```python
from build123d import *

# Parameters (mm, degrees)
F0_R     = 15
F1_DEPTH = 1.5
F2_DEPTH = 6.8


with BuildPart() as f1:
    # F0 (on Top) → F1 (new body)
    with BuildSketch(Plane.XY):
        with BuildLine():
            ThreePointArc((24.1652138662, -4.8646622494), (24.5285040494, -2.4443790825), (24.65, 0))
            ThreePointArc((24.65, 0), (18.0037803541, 16.8370541652), (1.6490756219, 24.5947768763))
            ThreePointArc((1.6490756219, 24.5947768763), (0, 23), (-1.6490756219, 24.5947768763))
            ThreePointArc((-1.6490756219, 24.5947768763), (-17.4301821562, 17.4301821562), (-24.5947768763, 1.6490756219))
            ThreePointArc((-24.5947768763, 1.6490756219), (-23.4639101733, 1.1470357113), (-23, 0))
            ThreePointArc((-23, 0), (-23.4639101733, -1.1470357113), (-24.5947768763, -1.6490756219))
            ThreePointArc((-24.5947768763, -1.6490756219), (-17.9529932576, -16.8911969112), (-3.1435634706, -24.4487322515))
            ThreePointArc((-3.1435634706, -24.4487322515), (0, -21.5), (3.1435634706, -24.4487322515))
            Line((3.1435634706, -24.4487322515), (12.969203616, -16.0692954907))
            ThreePointArc((12.969203616, -16.0692954907), (-18.6311104697, 8.9052918349), (20.65, 0))
            ThreePointArc((20.65, 0), (19.4738226895, -6.8696964896), (16.0792755585, -12.9568282197))
            Line((16.0792755585, -12.9568282197), (24.1652138662, -4.8646622494))
        make_face()
        with BuildLine():
            ThreePointArc((1.6490756219, 24.5947768763), (18.0037803541, 16.8370541652), (24.65, 0))
            ThreePointArc((24.65, 0), (24.5285040494, -2.4443790825), (24.1652138662, -4.8646622494))
            Line((24.1652138662, -4.8646622494), (27.771636901, -1.2554616043))
            ThreePointArc((27.771636901, -1.2554616043), (27.7929083207, -0.6278909749), (27.8, 0))
            ThreePointArc((27.8, 0), (25.6818028962, 10.6435426433), (19.65, 19.6651341211))
            ThreePointArc((19.65, 19.6651341211), (-25.6858981613, 10.6336557988), (7.1e-09, -27.8))
            ThreePointArc((7.1e-09, -27.8), (-2.2974435124, -26.8050529709), (-3.1435634706, -24.4487322515))
            ThreePointArc((-3.1435634706, -24.4487322515), (-17.9529932576, -16.8911969112), (-24.5947768763, -1.6490756219))
            ThreePointArc((-24.5947768763, -1.6490756219), (-26.3, 0), (-24.5947768763, 1.6490756219))
            ThreePointArc((-24.5947768763, 1.6490756219), (-17.4301821562, 17.4301821562), (-1.6490756219, 24.5947768763))
            ThreePointArc((-1.6490756219, 24.5947768763), (-0.0276154299, 26.2997688893), (1.65, 24.65))
            ThreePointArc((1.65, 24.65), (1.6497688893, 24.6223845701), (1.6490756219, 24.5947768763))
        make_face()
        with BuildLine():
            ThreePointArc((3.15, -24.65), (3.1483904564, -24.549314679), (3.1435634706, -24.4487322515))
            ThreePointArc((3.1435634706, -24.4487322515), (2.3974318813, -24.5331371898), (1.6490756219, -24.5947768763))
            ThreePointArc((1.6490756219, -24.5947768763), (1.6497688893, -24.6223845701), (1.65, -24.65))
            ThreePointArc((1.65, -24.65), (-0.0276154299, -26.2997688893), (-1.6490756219, -24.5947768763))
            ThreePointArc((-1.6490756219, -24.5947768763), (-2.3974318813, -24.5331371898), (-3.1435634706, -24.4487322515))
            ThreePointArc((-3.1435634706, -24.4487322515), (-2.2974435124, -26.8050529709), (7.1e-09, -27.8))
            ThreePointArc((7.1e-09, -27.8), (2.2273863633, -26.8773863582), (3.15, -24.65))
        make_face()
        with BuildLine():
            ThreePointArc((1.6490756219, -24.5947768763), (2.3974318813, -24.5331371898), (3.1435634706, -24.4487322515))
            ThreePointArc((3.1435634706, -24.4487322515), (0, -21.5), (-3.1435634706, -24.4487322515))
            ThreePointArc((-3.1435634706, -24.4487322515), (-2.3974318813, -24.5331371898), (-1.6490756219, -24.5947768763))
            ThreePointArc((-1.6490756219, -24.5947768763), (0, -23), (1.6490756219, -24.5947768763))
        make_face()
        with BuildLine():
            Line((12.969203616, -16.0692954907), (16.0792755585, -12.9568282197))
            ThreePointArc((16.0792755585, -12.9568282197), (19.4738226895, -6.8696964896), (20.65, 0))
            ThreePointArc((20.65, 0), (-18.6311104697, 8.9052918349), (12.969203616, -16.0692954907))
        make_face()
        Circle(F0_R, mode=Mode.SUBTRACT)
        with BuildLine():
            ThreePointArc((27.8, 0), (27.7929083207, -0.6278909749), (27.771636901, -1.2554616043))
            Line((27.771636901, -1.2554616043), (34.1742395873, 5.1520722659))
            Line((34.1742395873, 5.1520722659), (19.65, 19.6651341211))
            ThreePointArc((19.65, 19.6651341211), (25.6818028962, 10.6435426433), (27.8, 0))
        make_face()
    extrude(amount=-F1_DEPTH)

    # F0 (on Top) → F2 (join)
    with BuildSketch(Plane.XY):
        with BuildLine():
            ThreePointArc((24.1652138662, -4.8646622494), (24.5285040494, -2.4443790825), (24.65, 0))
            ThreePointArc((24.65, 0), (18.0037803541, 16.8370541652), (1.6490756219, 24.5947768763))
            ThreePointArc((1.6490756219, 24.5947768763), (0, 23), (-1.6490756219, 24.5947768763))
            ThreePointArc((-1.6490756219, 24.5947768763), (-17.4301821562, 17.4301821562), (-24.5947768763, 1.6490756219))
            ThreePointArc((-24.5947768763, 1.6490756219), (-23.4639101733, 1.1470357113), (-23, 0))
            ThreePointArc((-23, 0), (-23.4639101733, -1.1470357113), (-24.5947768763, -1.6490756219))
            ThreePointArc((-24.5947768763, -1.6490756219), (-17.9529932576, -16.8911969112), (-3.1435634706, -24.4487322515))
            ThreePointArc((-3.1435634706, -24.4487322515), (0, -21.5), (3.1435634706, -24.4487322515))
            Line((3.1435634706, -24.4487322515), (12.969203616, -16.0692954907))
            ThreePointArc((12.969203616, -16.0692954907), (-18.6311104697, 8.9052918349), (20.65, 0))
            ThreePointArc((20.65, 0), (19.4738226895, -6.8696964896), (16.0792755585, -12.9568282197))
            Line((16.0792755585, -12.9568282197), (24.1652138662, -4.8646622494))
        make_face()
        with BuildLine():
            ThreePointArc((1.6490756219, 24.5947768763), (18.0037803541, 16.8370541652), (24.65, 0))
            ThreePointArc((24.65, 0), (24.5285040494, -2.4443790825), (24.1652138662, -4.8646622494))
            Line((24.1652138662, -4.8646622494), (27.771636901, -1.2554616043))
            ThreePointArc((27.771636901, -1.2554616043), (27.7929083207, -0.6278909749), (27.8, 0))
            ThreePointArc((27.8, 0), (25.6818028962, 10.6435426433), (19.65, 19.6651341211))
            ThreePointArc((19.65, 19.6651341211), (-25.6858981613, 10.6336557988), (7.1e-09, -27.8))
            ThreePointArc((7.1e-09, -27.8), (-2.2974435124, -26.8050529709), (-3.1435634706, -24.4487322515))
            ThreePointArc((-3.1435634706, -24.4487322515), (-17.9529932576, -16.8911969112), (-24.5947768763, -1.6490756219))
            ThreePointArc((-24.5947768763, -1.6490756219), (-26.3, 0), (-24.5947768763, 1.6490756219))
            ThreePointArc((-24.5947768763, 1.6490756219), (-17.4301821562, 17.4301821562), (-1.6490756219, 24.5947768763))
            ThreePointArc((-1.6490756219, 24.5947768763), (-0.0276154299, 26.2997688893), (1.65, 24.65))
            ThreePointArc((1.65, 24.65), (1.6497688893, 24.6223845701), (1.6490756219, 24.5947768763))
        make_face()
        with BuildLine():
            ThreePointArc((3.15, -24.65), (3.1483904564, -24.549314679), (3.1435634706, -24.4487322515))
            ThreePointArc((3.1435634706, -24.4487322515), (2.3974318813, -24.5331371898), (1.6490756219, -24.5947768763))
            ThreePointArc((1.6490756219, -24.5947768763), (1.6497688893, -24.6223845701), (1.65, -24.65))
            ThreePointArc((1.65, -24.65), (-0.0276154299, -26.2997688893), (-1.6490756219, -24.5947768763))
            ThreePointArc((-1.6490756219, -24.5947768763), (-2.3974318813, -24.5331371898), (-3.1435634706, -24.4487322515))
            ThreePointArc((-3.1435634706, -24.4487322515), (-2.2974435124, -26.8050529709), (7.1e-09, -27.8))
            ThreePointArc((7.1e-09, -27.8), (2.2273863633, -26.8773863582), (3.15, -24.65))
        make_face()
        with BuildLine():
            ThreePointArc((1.6490756219, -24.5947768763), (2.3974318813, -24.5331371898), (3.1435634706, -24.4487322515))
            ThreePointArc((3.1435634706, -24.4487322515), (0, -21.5), (-3.1435634706, -24.4487322515))
            ThreePointArc((-3.1435634706, -24.4487322515), (-2.3974318813, -24.5331371898), (-1.6490756219, -24.5947768763))
            ThreePointArc((-1.6490756219, -24.5947768763), (0, -23), (1.6490756219, -24.5947768763))
        make_face()
        with BuildLine():
            ThreePointArc((27.8, 0), (27.7929083207, -0.6278909749), (27.771636901, -1.2554616043))
            Line((27.771636901, -1.2554616043), (34.1742395873, 5.1520722659))
            Line((34.1742395873, 5.1520722659), (19.65, 19.6651341211))
            ThreePointArc((19.65, 19.6651341211), (25.6818028962, 10.6435426433), (27.8, 0))
        make_face()
    extrude(amount=F2_DEPTH)


solid = f1.part
```
Input: part model. Units: mm. Frame: model coordinates. Give positions to 0.01 mm unless a question says otherwise; leave off trailing zeros. Order: outer loops, then holes, each group sorted by start corner. A loop starts at its lowest first (then second) coordinate and runs counter-clockwise, first axis right, second up. Notation, with made-up numbers: M -2.75,64.25 L 19.25,64.25 A21 cw 19.25,81.25 Z; hole C -37.75,19 d3. An arc over 180 degrees is marked long. Return JSON: item names as keys, results as strings.
Item 1: Cut plane D-D (y = 17). Return loops of the section in (x, z), then the cut area to 3 significant figures.
Solutions:
{"outline": "M -22,-1.5 L 22.32,-1.5 L 22.32,6.8 L 11.72,6.8 L 11.72,0 L -11.72,0 L -11.72,6.8 L -22,6.8 Z", "area": "208 mm^2"}
Item 2: Cut plane A-A (z = 5.5). Return loops of the section in (x, y), then the cut area to 3 significant figures.
Solutions:
{"outline": "M 0,-27.8 A3.15 ccw 3.14,-24.45 L 12.97,-16.07 A20.65 cw long 16.08,-12.96 L 34.17,5.15 L 19.65,19.67 A27.8 ccw long Z; hole C -24.65,0 d3.3; hole C 0,-24.65 d3.3; hole C 0,24.65 d3.3", "area": "926 mm^2"}
Item 3: Pull-direction query (Y, two-part tool) for faces 1 (the cylindrical face through (-14.985, 0.66, -0.74)), 2 (the cylindrical face through (-25.4, 11.3, 2.6)), 3 (the flat face through (14, 6, 0)), 4 (the flat face through (7.988, -20.318, 2.592)); classes: +Y half, -Y half, draft (parallel to the pull), parting line (faces both ways), or undercut.
Solutions:
{"face 1": "undercut", "face 2": "parting line", "face 3": "undercut", "face 4": "-Y half"}
Item 4: First-contact query: P1, Ø5, axis at x = -6.5, y = 13, coming from the +Z side; P2, Ø18, axis at x = 0, y = 0, coming from the +Z side; P3, Ø1, axis at x = 7, z = 0, coming from the +Y side; P4, Ø2, axis at y = 18.5, z = 3.5, coming from the -X side. Flat tips, straight axial feed; report the tip coordinate or a pass-through.
Solutions:
{"P1": "z = 0", "P2": "through", "P3": "y = 27.03", "P4": "x = -21.6"}
Item 5: Cut plane B-B (x = -4). Return loops of the section in (y, z), then the cut area to 3 significant figures.
Solutions:
{"outline": "M -27.51,-1.5 L -14.46,-1.5 L -14.46,0 L -20.26,0 L -20.26,6.8 L -27.51,6.8 Z; M 14.46,-1.5 L 27.51,-1.5 L 27.51,6.8 L 20.26,6.8 L 20.26,0 L 14.46,0 Z", "area": "138 mm^2"}
Item 6: Cut plane C-C (y = -6). Return loops of the section in (x, z), then the cut area to 3 significant figures.
Solutions:
{"outline": "M -27.14,-1.5 L -13.75,-1.5 L -13.75,0 L -19.76,0 L -19.76,6.8 L -27.14,6.8 Z; M 13.75,-1.5 L 23.03,-1.5 L 23.03,6.8 L 19.76,6.8 L 19.76,0 L 13.75,0 Z", "area": "106 mm^2"}
Item 7: Ray query, probe 1 along X at (y, z) = (-1.5, 3); probe 2 along Z at (x, y) = (13, -12); probe 3 along Y at (x, z) = (0.5, 1). Return the intervals inside material, ascending.
Solutions:
{"probe 1": "-27.76 to -25.34, -23.96 to -20.6, 20.6 to 27.53", "probe 2": "-1.5 to 0", "probe 3": "-27.76 to -26.22, -23.08 to -20.64, 20.64 to 23.08, 26.22 to 27.8"}
